Verification items for the finished model (mm, model axes). Face numbers are marked on the shaded views. A direction names the side the tool comes from. Round coordinates to 2 decimals unless told otherwise and drop trailing zeros. Write each loop counter-clockwise with the first axis right and the second up, starting at its lowest first coordinate (ties: lowest second). Pieces come first, ordered by that corner, then holes. Notation, with made-up numbers: (-7, -37.75) - (6, -37.75) arc R30 ccw to (6, -2.75) - close; hole circle Ø6 at (-39.75, -22.75). An arc over 180 degrees is marked (long way). Answer as a JSON object with one key per item and string values.
```python
from build123d import *

# Parameters (mm, degrees)
SKETCH1_W               = 15
SKETCH1_H               = 40
BOSS_EXTRUDE1_DEPTH     = 130
SKETCH2_W               = 15
SKETCH2_H               = 117.5
CUT_EXTRUDE1_DEPTH      = 30
CUT_EXTRUDE2_DEPTH      = 133.594306062
CUT_EXTRUDE2_DEPTH_BACK = 133.594306062
SKETCH3_R               = 1.5


with BuildPart() as part:
    # Sketch1 → Boss-Extrude1 (new body)
    with BuildSketch(Plane.XY):
        with Locations((0, 5)):
            Rectangle(SKETCH1_W, SKETCH1_H)
    extrude(amount=BOSS_EXTRUDE1_DEPTH)

    # Sketch2 → Cut-Extrude1 (cut)
    with BuildSketch(Plane(origin=(0, 25, 0), x_dir=(1, 0, 0), z_dir=(0, 1, 0))):
        with Locations((0, -65)):
            Rectangle(SKETCH2_W, SKETCH2_H)
    extrude(amount=-CUT_EXTRUDE1_DEPTH, mode=Mode.SUBTRACT)

    # Sketch3 → Cut-Extrude2 (cut, two sides: drawn at the far end of the back side and taken through both)
    with BuildSketch(Plane(origin=(0, 0, 0), x_dir=(-1, 0, 0), z_dir=(0, 0, -1)).offset(-CUT_EXTRUDE2_DEPTH_BACK)):
        with Locations((0.28935703, 16.716588701)):
            Circle(SKETCH3_R)
        with Locations((0.28935703, -3.283411299)):
            Circle(SKETCH3_R)
    extrude(amount=CUT_EXTRUDE2_DEPTH + CUT_EXTRUDE2_DEPTH_BACK, mode=Mode.SUBTRACT)


solid = part.part
```
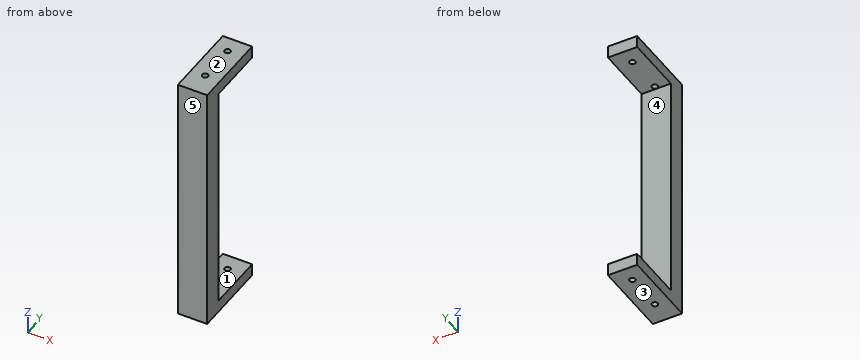
Q1. Release check for a two-part mould opening along Z. For the marked faces 3, 4 and 5 record: released by +Z, released by -Z, zero draft, split by the parting line, or undercut.
Geometry check:
{"face 3": "released by -Z", "face 4": "undercut", "face 5": "zero draft"}
Q2. Section check A-A, the plane y = 0. Record the cut outline in (x, z), then the cut area to 4 significant figures.
Geometry check:
{"outline": "(-7.5, 0) - (7.5, 0) - (7.5, 6.25) - (-7.5, 6.25) - close; (-7.5, 123.75) - (7.5, 123.75) - (7.5, 130) - (-7.5, 130) - close", "area": "187.5 mm2"}
Q3. Section check B-B, the plane x = -0.5. Record the cut outline in (y, z), then the cut area to 3 significant figures.
Geometry check:
{"outline": "(-15, 0) - (-4.77, 0) - (-4.77, 6.25) - (-5, 6.25) - (-5, 123.75) - (-4.77, 123.75) - (-4.77, 130) - (-15, 130) - close; (-1.8, 0) - (15.23, 0) - (15.23, 6.25) - (-1.8, 6.25) - close; (-1.8, 123.75) - (15.23, 123.75) - (15.23, 130) - (-1.8, 130) - close; (18.2, 0) - (25, 0) - (25, 6.25) - (18.2, 6.25) - close; (18.2, 123.75) - (25, 123.75) - (25, 130) - (18.2, 130) - close", "area": "1,600 mm2"}
Q4. Set-up check for the marked faces 1 and 2: record each of +Z, -Z, +X, -X, +Y, -Y from which the full face is reachable in a straight line by a thin tool's end or side.
Geometry check:
{"face 1": "+X, -X, +Y", "face 2": "+Z, +X, -X, +Y, -Y"}
Q5. Gauge pin test, flat ends, axial feed: P1, Ø6, axis at y = -3, z = 103, coming from the +X side; P2, Ø4.5, axis at x = 3.5, z = 86.5, coming from the +Y side; P3, Ø2.5, axis at x = -0.29, y = 16.72, coming from the -Z side (3 decimals). Record the tip position at first contact, or that the pin passes through.
Geometry check:
{"P1": "stops at x = 7.5", "P2": "stops at y = -5", "P3": "passes through"}
Q6. Material ranges on line 1 along Z through (x, y) = (2.5, 12.5); line 2 along Y through (x, z) = (5.5, 110.5), recorded low to high. Write a range as [from, to].
Geometry check:
{"line 1": "z = [0, 6.25], [123.75, 130]", "line 2": "y = [-15, -5]"}
Q7. Section check C-C, the plane z = 110. Record the cut outline in (x, y).
Geometry check:
{"outline": "(-7.5, -15) - (7.5, -15) - (7.5, -5) - (-7.5, -5) - close"}
